from build123d import *

# Parameters (mm, degrees)
F0_W     = 42.545
F0_H     = 165.1
F1_DEPTH = 25.4
F2_W     = 39.37
F2_H     = 161.925
F3_DEPTH = 22.225
F4_W     = 39.37
F4_H     = 15.24
F5_DEPTH = 3.175
F6_W     = 50.8
F6_H     = 5.08
F7_DEPTH = 6.35
F8_W     = 6.35
F8_H     = 25.4
F9_DEPTH = 3.176
F10_R    = 5.08


with BuildPart() as f1:
    # F0 (on Top) → F1 (new body)
    with BuildSketch(Plane.XY):
        with Locations((-43.306965, -1.745749)):
            Rectangle(F0_W, F0_H)
    extrude(amount=F1_DEPTH)

    # F2 (on face) → F3 (cut)
    with BuildSketch(Plane.XY.offset(25.4)):
        with Locations((-41.719465, -0.158249)):
            Rectangle(F2_W, F2_H)
    extrude(amount=-F3_DEPTH, mode=Mode.SUBTRACT)

    # F4 (on face) → F5 (join)
    with BuildSketch(Plane.XY.offset(25.4)):
        with Locations((-41.719465, -73.500749)):
            Rectangle(F4_W, F4_H)
    extrude(amount=-F5_DEPTH)

    # F6 (on face) → F7 (join)
    with BuildSketch(Plane.YZ.offset(-61.404465)):
        with Locations((45.879251, 10.795)):
            Rectangle(F6_W, F6_H)
    extrude(amount=F7_DEPTH)

    # F8 (on face) → F9 (cut, through all)
    with BuildSketch(Plane.XY.offset(3.175)):
        with Locations((-25.209465, -58.895749)):
            Rectangle(F8_W, F8_H)
        with Locations((-25.209465, -8.095749)):
            Rectangle(F8_W, F8_H)
        with Locations((-25.209465, 42.704251)):
            Rectangle(F8_W, F8_H)
    extrude(amount=-F9_DEPTH, mode=Mode.SUBTRACT)

    # F10
    f10_edges = [f1.edges().sort_by_distance(p)[0] for p in [
        (-64.579465, -84.295749, 12.7),
    ]]
    fillet(f10_edges, radius=F10_R)


solid = f1.part
Verification items for the finished model (mm, model axes). A direction names the side the tool comes from. Coordinates: 2 decimals unless noted, no trailing zeros. Write each loop counter-clockwise with the first axis right and the second up, starting at its lowest first coordinate (ties: lowest second). Pieces come first, ordered by that corner, then holes. Notation, with made-up numbers: (-29.5, 86.5) - (-25.5, 86.5) arc R29 ccw to (-25.5, 111.5) - close; hole circle Ø10 at (-1, 87). An arc over 180 degrees is marked (long way). Answer as a JSON object with one key per item and string values.
(1) Cross-section at C-C on x = -32.5. Record the cut outline in (y, z) (3 decimals), plus the area to 3 significant figures.
Report:
{"outline": "(-84.296, 0) - (80.804, 0) - (80.804, 3.175) - (-81.121, 3.175) - (-81.121, 22.225) - (-65.881, 22.225) - (-65.881, 25.4) - (-84.296, 25.4) - close", "area": "643 mm^2"}
(2) Thickness scan on line 1 along Z through (x, y) = (-61, 41) (3 decimals); line 2 along Z through (x, y) = (-39.5, -70) (3 decimals); line 3 along X through (y, z) = (-64, 10.5). Record the ranges inside material, lowest first.
Report:
{"line 1": "0 to 3.175, 8.255 to 13.335", "line 2": "0 to 3.175, 22.225 to 25.4", "line 3": "-64.58 to -61.4"}
(3) Cross-section at D-D on z = 11.5. Record the cut outline in (x, y).
Report:
{"outline": "(-64.58, -79.22) arc R5.08 ccw to (-59.5, -84.3) - (-22.03, -84.3) - (-22.03, -81.12) - (-61.4, -81.12) - (-61.4, 20.48) - (-55.05, 20.48) - (-55.05, 71.28) - (-61.4, 71.28) - (-61.4, 80.8) - (-64.58, 80.8) - close"}
(4) Gauge pin test, flat ends, axial feed: pin 1 Ø5 at (x, y) = (-58.5, 41.5) entering from +Z (3 decimals); pin 2 Ø4 at (x, z) = (-49.5, 9.5) entering from +Y; pin 3 Ø8 at (y, z) = (37.5, 21.5) entering from +X. Record the tip position at first contact, or that the pin passes through.
Report:
{"pin 1": "z = 13.335", "pin 2": "y = -81.12", "pin 3": "x = -61.4"}
(5) Tool access check on faces 1 (the flat face through (-42, 1, 3.175)), 2 (the flat face through (-58, 20.479, 11)), 3 (the flat face through (-55.054, 46, 11)). Record the directions out of +Z, -Z, +X, -X, +Y, -Y that give a thin tool (end or side, any length) a straight path to the whole face; none if there is none.
Report:
{"face 1": "+X, +Y", "face 2": "+Z, +X", "face 3": "+Z, +X, +Y"}
(6) Mould release check, pull along Z, two halves, no side actions. Record for faces 4 (the flat face through (-44, -1, 0)), 5 (the flat face through (-28.384, 43, 2)), 6 (the flat face through (-61.404, -1, 14)): pulls with the +Z half, pulls with the -Z half, needs draft (parallel to the pull), parting line crosses it, or undercut.
Report:
{"face 4": "pulls with the -Z half", "face 5": "needs draft", "face 6": "undercut"}
(7) Cross-section at A-A on z = 19. Record the cut outline in (x, y).
Report:
{"outline": "(-64.58, -79.22) arc R5.08 ccw to (-59.5, -84.3) - (-22.03, -84.3) - (-22.03, -81.12) - (-61.4, -81.12) - (-61.4, 80.8) - (-64.58, 80.8) - close"}
(8) Cross-section at B-B on y = 32.5. Record the cut outline in (x, z) (3 decimals).
Report:
{"outline": "(-64.579, 0) - (-28.384, 0) - (-28.384, 3.175) - (-61.404, 3.175) - (-61.404, 8.255) - (-55.054, 8.255) - (-55.054, 13.335) - (-61.404, 13.335) - (-61.404, 25.4) - (-64.579, 25.4) - close"}
